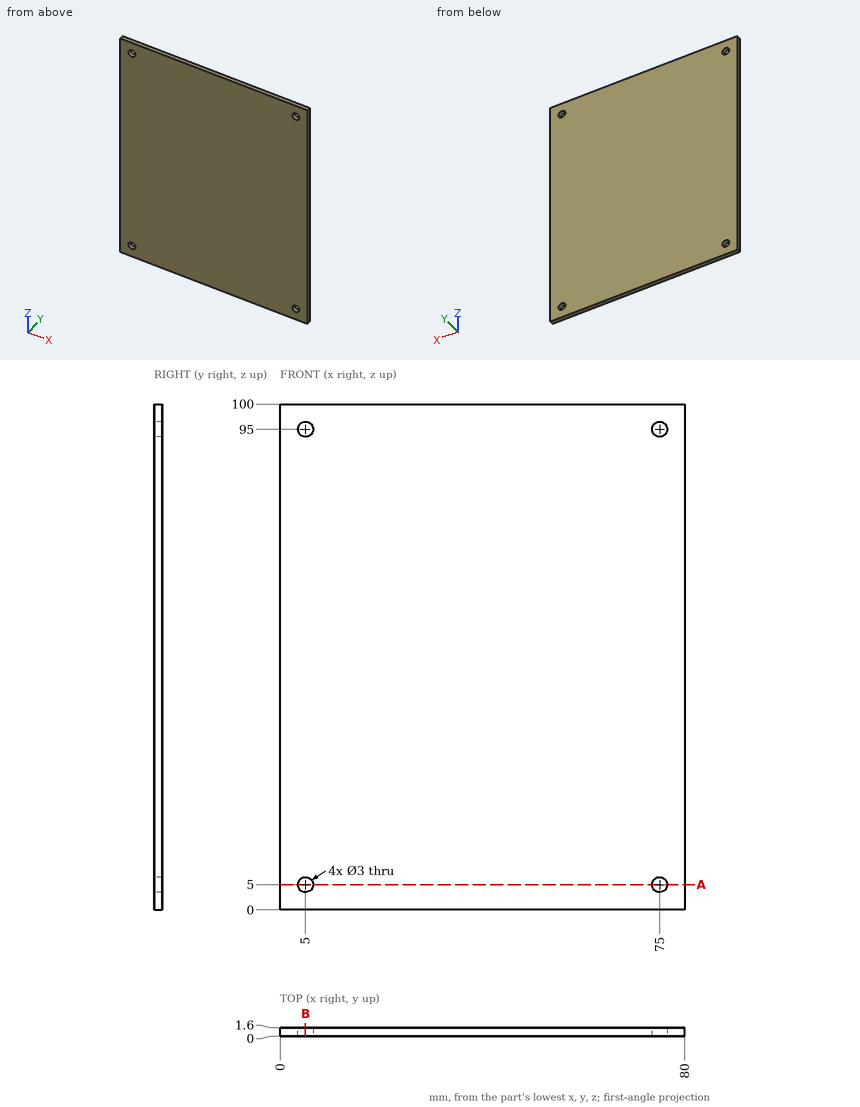
Geometry check sheet. Reference: drawing and pictorial views, mm from the part's lowest x, y, z. Round coordinates to 2 decimals unless told otherwise and drop trailing zeros. Loops run counter-clockwise (first coordinate to the right, second up) from the corner with the lowest first, then second, coordinate; pieces in that order, holes last. Notation, with made-up numbers: M 66,49.25 L 103,49.25 A15 cw 103,60.25 Z; hole C 58,-23 d8. An arc over 180 degrees is marked long. Return JSON: item names as keys, results as strings. Group by question number.
(1) Section check A-A, the plane z = 5. Enter the section's corners in (x, y), and give its area (3 significant figures).
(2) Section check B-B, the plane x = 5. Enter the section's corners in (y, z), and give its area (3 significant figures).
(3) Scan lines: line 1 along Z through (x, y) = (5, 0.55); line 2 along Z through (x, y) = (74.5, 0.15); line 3 along X through (y, z) = (0.3, 94.5). Record each from-to range of solid material in increasing order. Write a range as [from, to].
(4) Go/stop test with a flat-tipped pin: pin 1 (1.8 mm diameter, centred on x = 75, z = 95, fed in from -Y) (3 decimals). Record where the tip stops, or that it passes through.
Data:
{
 "1": {"outline": "M 0,0 L 3.5,0 L 3.5,1.6 L 0,1.6 Z; M 6.5,0 L 73.5,0 L 73.5,1.6 L 6.5,1.6 Z; M 76.5,0 L 80,0 L 80,1.6 L 76.5,1.6 Z", "area": "118 mm²"},
 "2": {"outline": "M 0,0 L 1.6,0 L 1.6,3.5 L 0,3.5 Z; M 0,6.5 L 1.6,6.5 L 1.6,93.5 L 0,93.5 Z; M 0,96.5 L 1.6,96.5 L 1.6,100 L 0,100 Z", "area": "150 mm²"},
 "3": {"line 1": "[0, 3.5], [6.5, 93.5], [96.5, 100]", "line 2": "[0, 3.59], [6.41, 93.59], [96.41, 100]", "line 3": "[0, 3.59], [6.41, 73.59], [76.41, 80]"},
 "4": {"pin 1": "through"}
}
